```python
from build123d import *

# Parameters (mm, degrees)
PAD_DEPTH    = 3.5
SKETCH001_R  = 1
PAD001_DEPTH = 1.5
FILLET_R     = 1


with BuildPart() as part:
    # Sketch → Pad (new body, symmetric)
    with BuildSketch(Plane.XY):
        Polygon((0, 0), (15, 0), (15, -3), (11.5, -3), (11.5, -5), (17, -5), (17, 2), (-17, 2), (-17, -5), (-11.5, -5), (-11.5, -3), (-15, -3), (-15, 0), align=None)
    extrude(amount=PAD_DEPTH, both=True)

    # Sketch001 (on Face11 of Pad) → Pad001 (join)
    with BuildSketch(Plane(origin=(0, -3, 0), x_dir=(-1, 0, 0), z_dir=(0, 1, 0))):
        with Locations((-13, 0)):
            Circle(SKETCH001_R)
        with Locations((13, 0)):
            Circle(SKETCH001_R)
    extrude(amount=PAD001_DEPTH)

    # Fillet
    fillet_edges = [part.edges().sort_by_distance(p)[0] for p in [
        (14.25, -5, 3.5),
        (-14.25, -5, 3.5),
        (-14.25, -5, -3.5),
        (14.25, -5, -3.5),
        (-17, -1.5, 3.5),
        (17, -1.5, 3.5),
        (17, -1.5, -3.5),
        (-17, -1.5, -3.5),
    ]]
    fillet(fillet_edges, radius=FILLET_R)


solid = part.part
```
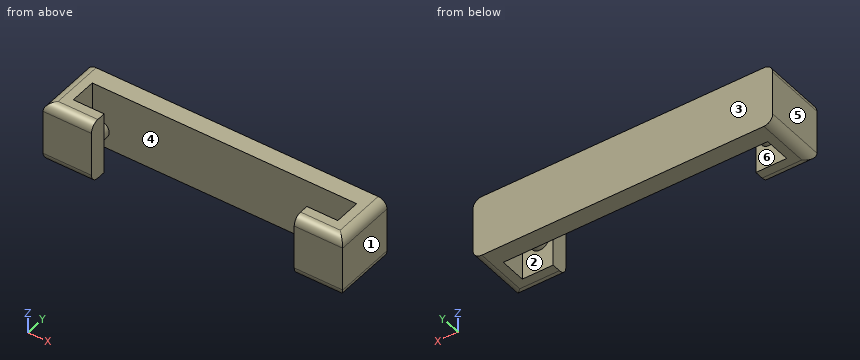
Source: CAD feature listing. Evaluate the final solid. Frame: model axes, mm. Face numbers are marked on the shaded views. A direction names the side the tool comes from. Round coordinates to 2 decimals unless told otherwise and drop trailing zeros. Loops run counter-clockwise (first coordinate to the right, second up) from the corner with the lowest first, then second, coordinate; pieces in that order, holes last.
(1) Material intervals for probe 1 along X at (y, z) = (-0.5, 2); probe 2 along X at (y, z) = (-3.75, -2.5); probe 3 along Y at (x, z) = (14, 2.5), sorted ascending.
From the geometry:
probe 1: x = -17 to -15, 15 to 17
probe 2: x = -17 to -11.5, 11.5 to 17
probe 3: y = -5 to -3, 0 to 2
(2) Pull-direction query (X, two-part tool) for the marked faces 1, 2 and 3; classes: +X half, -X half, draft (parallel to the pull), parting line (faces both ways), or undercut.
From the geometry:
face 1: +X half
face 2: undercut
face 3: draft
(3) Access query for the marked faces 4, 5 and 6. Directions: +Z, -Z, +X, -X, +Y, -Y. A direction counts if a zero-diameter tool reaches every point of the face in a straight line with its end or side. Return the directions, or none.
From the geometry:
face 4: +Z, -Z
face 5: +Z, -Z, -X, +Y, -Y
face 6: none
(4) Section query D-D (x = 10). Output: boundary loops of the cut face in (y, z), and give its area (3 significant figures).
From the geometry:
outline: (0, -3.5) - (2, -3.5) - (2, 3.5) - (0, 3.5) - close
area: 14.0 mm2
(5) Contact query for a flat-ended pin moving along its axis: pin 1 Ø4 at (x, z) = (0, 1.5) entering from -Y. Output: stop coordinate, or through.
From the geometry:
pin 1: stops at y = 0
(6) Section query A-A (x = -13). Output: boundary loops of the cut face in (y, z).
From the geometry:
outline: (-5, -2.5) arc R1 ccw to (-4, -3.5) - (-3, -3.5) - (-3, -1) - (-1.5, -1) - (-1.5, 1) - (-3, 1) - (-3, 3.5) - (-4, 3.5) arc R1 ccw to (-5, 2.5) - close; (0, -3.5) - (2, -3.5) - (2, 3.5) - (0, 3.5) - close
(7) Section query C-C (z = 0). Output: boundary loops of the cut face in (x, y), and give its area (3 significant figures).
From the geometry:
outline: (-17, -5) - (-11.5, -5) - (-11.5, -3) - (-12, -3) - (-12, -1.5) - (-14, -1.5) - (-14, -3) - (-15, -3) - (-15, 0) - (15, 0) - (15, -3) - (14, -3) - (14, -1.5) - (12, -1.5) - (12, -3) - (11.5, -3) - (11.5, -5) - (17, -5) - (17, 2) - (-17, 2) - close
area: 108 mm2
(8) Section query B-B (y = -2.5). Output: boundary loops of the cut face in (x, z), and give its area (3 significant figures).
From the geometry:
outline: (-17, -2.5) arc R1 ccw to (-16, -3.5) - (-15, -3.5) - (-15, 3.5) - (-16, 3.5) arc R1 ccw to (-17, 2.5) - close; circle Ø2 at (-13, 0); circle Ø2 at (13, 0); (15, -3.5) - (16, -3.5) arc R1 ccw to (17, -2.5) - (17, 2.5) arc R1 ccw to (16, 3.5) - (15, 3.5) - close
area: 33.4 mm2
